Source: CAD feature listing. Evaluate the final solid. Frame: model axes, mm. A direction names the side the tool comes from. Give positions to 0.01 mm unless a question says otherwise; leave off trailing zeros. Loops run counter-clockwise (first coordinate to the right, second up) from the corner with the lowest first, then second, coordinate; pieces in that order, holes last. Notation, with made-up numbers: M 15,76.5 L 41,76.5 A21 cw 41,103.5 Z; hole C 54,48.5 d9. An arc over 180 degrees is marked long. Put each result on its own line as item: value.
from build123d import *

# Parameters (mm, degrees)
EXTRUDE1_DEPTH     = 2.7
SKETCH4_R          = 1.5
CUT_EXTRUDE1_DEPTH = 7.759437846


with BuildPart() as part:
    # Sketch1 → Extrude1 (new body)
    with BuildSketch(Plane.XY.offset(1)):
        Polygon((0, 3.175426481), (-2.75, 1.58771324), (-2.75, -1.58771324), (0, -3.175426481), (2.75, -1.58771324), (2.75, 1.58771324), align=None)
    extrude(amount=EXTRUDE1_DEPTH)

    # Sketch2 → Revolve1 (revolve)
    with BuildSketch(Plane(origin=(0, 0, 0), x_dir=(0, 0, -1), z_dir=(1, 0, 0)), mode=Mode.PRIVATE) as revolve1_sk:
        with BuildLine():
            Line((0, 0), (0, 3))
            ThreePointArc((0, 3), (-0.292893219, 3.707106781), (-1, 4))
            Line((-1, 4), (-2.07179677, 0))
            Line((-2.07179677, 0), (0, 0))
        make_face()
    revolve(revolve1_sk.sketch.rotate(Axis((0, 0, 0), (0, 0, 1)), 90), axis=Axis((0, 0, 0), (0, 0, 1)))

    # Sketch3 → Cut-Revolve1 (revolve, cut)
    with BuildSketch(Plane(origin=(0, 0, 0), x_dir=(1, 0, 0), z_dir=(0, 1, 0))):
        Polygon((-2.75, -3.7), (-3.85, -3.7), (-3.85, -3.064914704), align=None)
    revolve(axis=Axis((0, 0, 0), (0, 0, 1)), mode=Mode.SUBTRACT)

    # Sketch4 → Cut-Extrude1 (cut, through all)
    with BuildSketch(Plane(origin=(0, 0, 0), x_dir=(-1, 0, 0), z_dir=(0, 0, -1))):
        Circle(SKETCH4_R)
    extrude(amount=-CUT_EXTRUDE1_DEPTH, mode=Mode.SUBTRACT)


solid = part.part
1. Access query for faces 1 (the flat face through (-1.36, 2.39, 2.44)), 2 (the flat face through (1.394, 2.37, 2.443)), 3 (the flat face through (1.36, -2.39, 2.44)). Directions: +Z, -Z, +X, -X, +Y, -Y. A direction counts if a zero-diameter tool reaches every point of the face in a straight line with its end or side. Return the directions, or none.
Found:
face 1: +Z, -X, +Y
face 2: +Z, +X, +Y
face 3: +Z, +X, -Y
2. Contact query for flat-ended pins moving along their axis: P1, Ø4, axis at x = 0, y = 0, coming from the +Z side; P2, Ø1.2, axis at y = 0, z = 3, coming from the +X side; P3, Ø2, axis at y = 0.5, z = 2.5, coming from the -X side. Output: stop coordinate, or through.
Found:
P1: z = 3.7
P2: x = 2.75
P3: x = -2.75
3. Material intervals for line 1 (X direction, y = 1, z = 3.3); line 2 (X direction, y = -0.75, z = 1.75); line 3 (Y direction, x = 1, z = 2.8), sorted ascending. Write a range as from..to.
Found:
line 1: -2.75..-1.12, 1.12..2.75
line 2: -2.75..-1.3, 1.3..2.75
line 3: -2.6..-1.12, 1.12..2.6
4. Section query A-A (z = 2.35). Output: boundary loops of the cut face in (x, y).
Found:
outline: M -2.75,-1.59 L 0,-3.18 L 2.75,-1.59 L 2.75,1.59 L 0,3.18 L -2.75,1.59 Z; hole C 0,0 d3
5. Draft query along X for faces 4 (the conical face through (2.95, -0.13, 1.28)), 5 (the flat face through (-1.394, -2.37, 2.443)), 6 (the cylindrical face through (1.5, 0.07, 1.82)). Return one class per face: pulls with the +X half, pulls with the -X half, needs draft (parallel to the pull), parting line crosses it, or undercut.
Found:
face 4: parting line crosses it
face 5: pulls with the -X half
face 6: undercut
